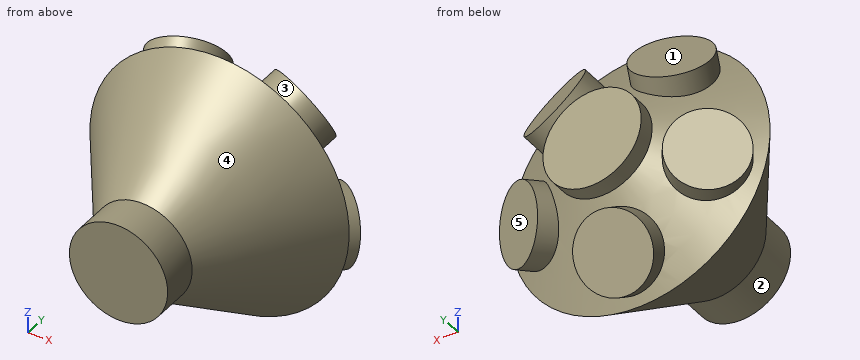
```python
from build123d import *

# Parameters (mm, degrees)
F_7_16_0_4375_DIAMETER_HOLE1_D         = 11.1125
F_7_16_START                           = 1.779676233
F_7_16_0_4375_DIAMETER_HOLE2_OUTLINE_R = 5.55625
F_7_16_0_4375_DIAMETER_HOLE2_DEPTH     = 24.355951698
CIRPATTERN1_COUNT                      = 5
SKETCH11_R                             = 7.62
BOSS_EXTRUDE1_DEPTH                    = 2.54
BOSS_EXTRUDE2_START                    = 2.54
SKETCH12_R                             = 7.62
BOSS_EXTRUDE2_DEPTH                    = 2.54
BOSS_EXTRUDE3_REACH                    = 52.922
SKETCH13_R                             = 5.87375
SKETCH13_R_2                           = 5.55625
CUT_EXTRUDE1_START                     = -3.182233
SKETCH14_R                             = 5.55625
CUT_EXTRUDE1_DEPTH                     = 0.642233
CIRPATTERN3_COUNT                      = 5


# Read off the part's stored shape, not the designer's step: 7/16 (0.4375) Diameter Hole2
with BuildPart() as part:
    # Sketch1 → Revolve1 (revolve)
    with BuildSketch(Plane.XY, mode=Mode.PRIVATE) as revolve1_sk:
        Polygon((0, 0), (0, 26.570129165), (7.62, 26.570129165), (20.103877155, 17.828824275), (7.62, 0), (7.62, -3.175), (0, -3.175), align=None)
    revolve(revolve1_sk.sketch.rotate(Axis((0, 0, 0), (0, 1, 0)), 90), axis=Axis((0, 0, 0), (0, 1, 0)))

    # 7/16 (0.4375) Diameter Hole1 (through all)
    with Locations(Plane(origin=(0, 26.570129165, 0), x_dir=(1, 0, 0), z_dir=(0, 1, 0))):
        with Locations((0, 0)):
            Hole(F_7_16_0_4375_DIAMETER_HOLE1_D / 2)

    # 7/16 (0.4375) Diameter Hole2 outline → 7/16 (0.4375) Diameter Hole2 (cut)
    with BuildSketch(Plane(origin=(0, 0, 0), x_dir=(1, 0, 0), z_dir=(0, 0.8191520442889911, -0.5735764363510472)).offset(F_7_16_START)):
        with Locations((0, -1.246142784)):
            Circle(F_7_16_0_4375_DIAMETER_HOLE2_OUTLINE_R)
    f_7_16_0_4375_diameter_hole2 = extrude(amount=F_7_16_0_4375_DIAMETER_HOLE2_DEPTH, mode=Mode.SUBTRACT)

    # CirPattern1: 7/16 (0.4375) Diameter Hole2 ×5 about axis
    cirpattern1_axis = Axis((0, 26.570129165, 0), (0, 1, 0))
    for i in range(1, CIRPATTERN1_COUNT):
        add(f_7_16_0_4375_diameter_hole2.rotate(cirpattern1_axis, i * 360 / CIRPATTERN1_COUNT), mode=Mode.SUBTRACT)

    # Sketch11 → Boss-Extrude1 (add)
    with BuildSketch(Plane(origin=(0, 26.570129165, 0), x_dir=(1, 0, 0), z_dir=(0, 1, 0))):
        with Locations(Location((0, 0, 0), (0, 0, 90))):
            Circle(SKETCH11_R)
    extrude(amount=BOSS_EXTRUDE1_DEPTH)

    # Sketch12 → Boss-Extrude2 (add)
    with BuildSketch(Plane.XZ.offset(3.175).offset(BOSS_EXTRUDE2_START)):
        with Locations(Location((0, 0, 0), (0, 0, 270))):
            Circle(SKETCH12_R)
    extrude(amount=-BOSS_EXTRUDE2_DEPTH)

    # Boss-Extrude3: up to this cone (the profile starts outside it)
    boss_extrude3_end = Plane(origin=(0, 22.5675805, 0), z_dir=(0, -1, 0)).offset(-9.338129106) * Cone(1.428e-06, 111.014569628, 77.733237505, align=(Align.CENTER, Align.CENTER, Align.MIN), mode=Mode.PRIVATE)
    # Sketch13 → Boss-Extrude3 (add, up to the surface)
    with BuildSketch(Plane(origin=(0, 23.489699353, -16.447664557), x_dir=(1, 0, 0), z_dir=(0, 0.8191520442889909, -0.5735764363510475)), mode=Mode.PRIVATE) as boss_extrude3_sk1:
        with Locations(Location((0, -1.246142784, 0), (0, 0, 270))):
            Circle(SKETCH13_R)
        with Locations(Location((0, -1.246142784, 0), (0, 0, 306))):
            Circle(SKETCH13_R_2, mode=Mode.SUBTRACT)
    boss_extrude3_tool1 = extrude(boss_extrude3_sk1.sketch, amount=-BOSS_EXTRUDE3_REACH, mode=Mode.PRIVATE) - boss_extrude3_end
    # Sketch13 → Boss-Extrude3 (add, up to the surface)
    with BuildSketch(Plane(origin=(0, 23.489699353, -16.447664557), x_dir=(1, 0, 0), z_dir=(0, 0.8191520442889909, -0.5735764363510475)), mode=Mode.PRIVATE) as boss_extrude3_sk2:
        with Locations(Location((0, -1.246142784, 0), (0, 0, 306))):
            Circle(SKETCH13_R_2)
    boss_extrude3_tool2 = extrude(boss_extrude3_sk2.sketch, amount=-BOSS_EXTRUDE3_REACH, mode=Mode.PRIVATE) - boss_extrude3_end
    boss_extrude3 = boss_extrude3_tool1.solids().sort_by_distance((0, 20.930704, -20.102289))[0] + boss_extrude3_tool2.solids().sort_by_distance((0, 24.204457, -15.426884))[0]
    add(boss_extrude3)

    # Sketch14 → Cut-Extrude1 (cut)
    with BuildSketch(Plane(origin=(0, 23.489699353, -16.447664557), x_dir=(1, 0, 0), z_dir=(0, 0.8191520442889909, -0.5735764363510475)).offset(CUT_EXTRUDE1_START)):
        with Locations(Location((0, -1.246142784, 0), (0, 0, 270))):
            Circle(SKETCH14_R)
    cut_extrude1 = extrude(amount=CUT_EXTRUDE1_DEPTH, mode=Mode.SUBTRACT)

    # CirPattern3: Boss-Extrude3, Cut-Extrude1 ×5 about axis
    cirpattern3_axis = Axis((0, 0, 0), (0, 1, 0))
    add([boss_extrude3.rotate(cirpattern3_axis, i * 360 / CIRPATTERN3_COUNT) for i in range(1, CIRPATTERN3_COUNT)])
    add([cut_extrude1.rotate(cirpattern3_axis, i * 360 / CIRPATTERN3_COUNT) for i in range(1, CIRPATTERN3_COUNT)], mode=Mode.SUBTRACT)


solid = part.part
```
Build history of the part. All positions in model axes, mm. Face numbers are marked on the shaded views. A direction names the side the tool comes from. Round coordinates to 2 decimals unless told otherwise and drop trailing zeros. Answer as CSV lines item,"result".
Q1. Drill centre lines: probe 1 along Y at (x, z) = (-4, 0.5) (3 decimals); probe 2 along Z at (x, y) = (0, 22.5); probe 3 along X at (y, z) = (18.5, 10.5). Where is each one in solid material? Low to high. Write a range as [from, to].
Report:
probe 1,"y = [-5.715, -3.175], [26.57, 29.11]"
probe 2,"z = [-17.86, -13.43], [-7.45, -5.56], [5.56, 13.43]"
probe 3,"x = [-16.01, -12.73], [-1.15, 1.15], [12.73, 16.01]"
Q2. Cut at A-A (x = -14). State how many separate pieces and enclosed holes the cut face has, and give its area (3 significant figures).
Report:
separate pieces,"2"
enclosed holes,"1"
area,"214 mm^2"
Q3. Drop flat-ended pins along their axis: pin 1 (1.5 mm diameter, centred on x = 13.5, y = 15, fed in from +Z); pin 2 (12 mm diameter, centred on x = -10.5, y = 9, fed in from +Z); pin 3 (3 mm diameter, centred on y = 20.5, z = 15.5, fed in from -X). Give the stop position or say it passes through.
Report:
pin 1,"stops at z = 13.18"
pin 2,"stops at z = 15.88"
pin 3,"stops at x = -13.85"
Q4. Pull direction Y, two halves, no side cores. Call the marked faces 3, 4 and 5: +Y half, -Y half, draft (parallel to the pull), parting line (faces both ways), or undercut.
Report:
face 3,"undercut"
face 4,"-Y half"
face 5,"+Y half"
Q5. Tool access for the marked faces 1 and 2: list every direction of +Z, -Z, +X, -X, +Y, -Y with a clear straight run to the whole face (end or side of a thin tool).
Report:
face 1,"+Z, -X, +Y"
face 2,"-Y"
